Design review of the part built by this model. Coordinates are the model's own, in mm. Coordinates: 2 decimals unless noted, no trailing zeros. Write each loop counter-clockwise with the first axis right and the second up, starting at its lowest first coordinate (ties: lowest second). Pieces come first, ordered by that corner, then holes. Notation, with made-up numbers: (26, -5.5) - (56, -5.5) arc R31 cw to (56, 33.5) - close; hole circle Ø7 at (56, 74). An arc over 180 degrees is marked (long way). Answer as a JSON object with one key per item and string values.
```python
from build123d import *

# Parameters (mm, degrees)
F0_W           = 300
F0_H           = 100
F1_DEPTH       = 15
F3_SIZE        = 15
F4_D           = 5.5
F4_CBORE_D     = 8
F4_CBORE_DEPTH = 5


with BuildPart() as f1:
    # F0 (on Front) → F1 (new body)
    with BuildSketch(Plane.XZ):
        with Locations((150, 50)):
            Rectangle(F0_W, F0_H)
    extrude(amount=-F1_DEPTH)

    # F3
    f3_edges = [f1.edges().sort_by_distance(p)[0] for p in [
        (0, 7.5, 100),
        (300, 7.5, 100),
    ]]
    chamfer(f3_edges, length=F3_SIZE)

    # F4 (through all)
    with Locations(Plane.XZ):
        with Locations((127.5, 35.5), (150, 58), (172.5, 35.5), (150, 13)):
            CounterBoreHole(F4_D / 2, F4_CBORE_D / 2, F4_CBORE_DEPTH)


solid = f1.part
```
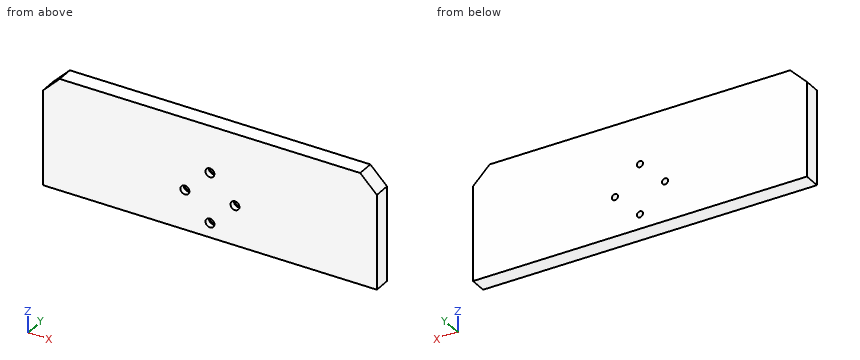
(1) For pin 1 (7 mm diameter, centred on x = 150, z = 13, fed in from -Y); pin 2 (3.5 mm diameter, centred on x = 150, z = 58, fed in from +Y), all flat-tipped, find the tip position at first contact; note any pin that passes through.
Solved:
{"pin 1": "stops at y = 5", "pin 2": "passes through"}
(2) Take a section at B-B, the plane x = 150. Write out the cut boundary in (y, z), and give its area (3 significant figures).
Solved:
{"outline": "(0, 0) - (15, 0) - (15, 10.25) - (5, 10.25) - (5, 9) - (0, 9) - close; (0, 17) - (5, 17) - (5, 15.75) - (15, 15.75) - (15, 55.25) - (5, 55.25) - (5, 54) - (0, 54) - close; (0, 62) - (5, 62) - (5, 60.75) - (15, 60.75) - (15, 100) - (0, 100) - close", "area": "1,310 mm^2"}
(3) Take a section at D-D, the plane z = 92. Write out the cut boundary in (x, y), and give its area (3 significant figures).
Solved:
{"outline": "(7, 0) - (293, 0) - (293, 15) - (7, 15) - close", "area": "4,290 mm^2"}
(4) To check wall thickness, follow line 1 (Z direction, x = 127.5, y = 9); line 2 (Z direction, x = 150, y = 2.2); line 3 (X direction, y = 7.25, z = 33). State the ranges of each line that lie inside material, in increasing order. Write a range as from..to.
Solved:
{"line 1": "z = 0..32.75, 38.25..100", "line 2": "z = 0..9, 17..54, 62..100", "line 3": "x = 0..126.35, 128.65..171.35, 173.65..300"}
(5) Take a section at A-A, the plane z = 58. Write out the cut boundary in (x, y).
Solved:
{"outline": "(0, 0) - (146, 0) - (146, 5) - (147.25, 5) - (147.25, 15) - (0, 15) - close; (152.75, 5) - (154, 5) - (154, 0) - (300, 0) - (300, 15) - (152.75, 15) - close"}
(6) Take a section at C-C, the plane z = 35.5. Write out the cut boundary in (x, y).
Solved:
{"outline": "(0, 0) - (123.5, 0) - (123.5, 5) - (124.75, 5) - (124.75, 15) - (0, 15) - close; (130.25, 5) - (131.5, 5) - (131.5, 0) - (168.5, 0) - (168.5, 5) - (169.75, 5) - (169.75, 15) - (130.25, 15) - close; (175.25, 5) - (176.5, 5) - (176.5, 0) - (300, 0) - (300, 15) - (175.25, 15) - close"}
